from build123d import *

# Parameters (mm, degrees)
F0_W     = 120
F0_H     = 40
F1_DEPTH = 12.5
F3_DEPTH = 9.7
F4_W     = 110
F4_H     = 10.5
F5_DEPTH = 30
F6_W     = 110
F6_H     = 1.62
F7_DEPTH = 3.6
F8_R     = 0.5


with BuildPart() as f1:
    # F0 (on Front) → F1 (new body)
    with BuildSketch(Plane.XZ):
        Rectangle(F0_W, F0_H)
    extrude(amount=F1_DEPTH)

    # F2 (on face) → F3 (join)
    with BuildSketch(Plane(origin=(0, 0, 0), x_dir=(-1, 0, 0), z_dir=(0, 1, 0))):
        with BuildLine():
            Line((-25, -10), (25, -10))
            ThreePointArc((25, -10), (28.5355339059, -8.5355339059), (30, -5))
            Line((30, -5), (30, 5))
            ThreePointArc((30, 5), (28.5355339059, 8.5355339059), (25, 10))
            Line((25, 10), (-25, 10))
            ThreePointArc((-25, 10), (-28.5355339059, 8.5355339059), (-30, 5))
            Line((-30, 5), (-30, -5))
            ThreePointArc((-30, -5), (-28.5355339059, -8.5355339059), (-25, -10))
        make_face()
    extrude(amount=F3_DEPTH)

    # F4 (on face) → F5 (cut)
    with BuildSketch(Plane(origin=(0, 0, -20), x_dir=(1, 0, 0), z_dir=(0, 0, -1))):
        with Locations((0, 7.25)):
            Rectangle(F4_W, F4_H)
    extrude(amount=-F5_DEPTH, mode=Mode.SUBTRACT)

    # F6 (on face) → F7 (join)
    with BuildSketch(Plane(origin=(0, 0, 10), x_dir=(1, 0, 0), z_dir=(0, 0, -1))):
        with Locations((0, 9.67)):
            Rectangle(F6_W, F6_H)
    extrude(amount=F7_DEPTH)

    # F8
    f8_edges = [f1.edges().sort_by_distance(p)[0] for p in [
        (0, 9.7, -10),
        (0, -2, -20),
        (55, -7.25, -20),
        (55, -12.5, -5),
        (0, -12.5, 10),
        (-55, -12.5, -5),
        (-55, -7.25, -20),
        (57.5, -12.5, -20),
        (60, -12.5, 0),
        (0, -12.5, 20),
        (-60, -12.5, 0),
        (-57.5, -12.5, -20),
        (60, -6.25, -20),
        (60, -6.25, 20),
        (-60, -6.25, 20),
        (-60, -6.25, -20),
        (-60, 0, 0),
        (0, 0, 20),
        (0, 0, -20),
        (60, 0, 0),
    ]]
    fillet(f8_edges, radius=F8_R)


solid = f1.part
The listing builds one solid part. Answer for the finished solid, in the listing's coordinates (mm). A direction names the side the tool comes from. Round coordinates to 2 decimals unless told otherwise and drop trailing zeros. Write each loop counter-clockwise with the first axis right and the second up, starting at its lowest first coordinate (ties: lowest second). Pieces come first, ordered by that corner, then holes. Notation, with made-up numbers: (81.25, 67.25) - (118.25, 67.25) arc R14 ccw to (118.25, 71.25) - close; hole circle Ø5 at (-39.5, 56). An arc over 180 degrees is marked (long way). Use one line per item in the form item = value. Start each with the question number.
Item 1: A cutting plane is placed at D-D (y = 2.5). Write down the section's boundary in (x, z).
Item 2: Determine the mould class of faces 5 (the cylindrical face through (-28, 5, -9)), 6 (the flat face through (60, -6, 0)), 7 (the flat face through (-55, -7, -5)) for opening direction X: +X half, -X half, draft (parallel to the pull), parting line (faces both ways), or undercut.
Item 3: A tool of negligible diameter and unlimited length cuts with its end or side. For faces 1 (the flat face through (0, 5, -10)), 2 (the flat face through (-30, 5, 0)), 3 (the flat face through (-1, -10.48, 8)), 4 (the flat face through (-1, -5, 10)), from which of +Z, -Z, +X, -X, +Y, -Y can it reach the whole face along a straight path? Write none if from no direction.
Item 4: A cutting plane is placed at A-A (y = -7). Write down the section's boundary in (x, z).
Item 5: A cutting plane is placed at B-B (z = -1.5). Write down the section's boundary in (x, y), plus the area to 3 significant figures.
Item 6: A cutting plane is placed at C-C (x = 46). Write down the section's boundary in (y, z), plus the area to 3 significant figures.
Item 7: Flat-ended cylindrical pins translate along their axes: pin 1 Ø0.5 at (x, y) = (-23, -11.5) entering from -Z; pin 2 Ø4 at (x, y) = (-11, 7) entering from -Z; pin 3 Ø6 at (y, z) = (5.5, -14) entering from +X; pin 4 Ø5 at (x, z) = (42.5, -4) entering from -Y. Find the tip coordinate at first contact, or state that the pin passes through.
Item 8: Find the intervals of material crossed by line 1 (X direction, y = -10, z = 6); line 2 (X direction, y = 1.5, z = 5); line 3 (Z direction, x = -24, y = 2), in increasing order. Write a range as [from, to].
The answers:
q1.outline = (-30, -5) arc R5 ccw to (-25, -10) - (25, -10) arc R5 ccw to (30, -5) - (30, 5) arc R5 ccw to (25, 10) - (-25, 10) arc R5 ccw to (-30, 5) - close
q2.face_5 = -X half
q2.face_6 = +X half
q2.face_7 = undercut
q3.face_1 = -Z, +X, -X, +Y
q3.face_2 = +Z, -Z, -X, +Y
q3.face_3 = -Z, -Y
q3.face_4 = -Z
q4.outline = (-60, -19.5) arc R0.5 ccw to (-59.5, -20) - (-55.5, -20) arc R0.5 ccw to (-55, -19.5) - (-55, 10) - (55, 10) - (55, -19.5) arc R0.5 ccw to (55.5, -20) - (59.5, -20) arc R0.5 ccw to (60, -19.5) - (60, 19.5) arc R0.5 ccw to (59.5, 20) - (-59.5, 20) arc R0.5 ccw to (-60, 19.5) - close
q5.outline = (-60, -12) arc R0.5 ccw to (-59.5, -12.5) - (-55.5, -12.5) arc R0.5 ccw to (-55, -12) - (-55, -2) - (55, -2) - (55, -12) arc R0.5 ccw to (55.5, -12.5) - (59.5, -12.5) arc R0.5 ccw to (60, -12) - (60, -0.5) arc R0.5 ccw to (59.5, 0) - (30, 0) - (30, 9.2) arc R0.5 ccw to (29.5, 9.7) - (-29.5, 9.7) arc R0.5 ccw to (-30, 9.2) - (-30, 0) - (-59.5, 0) arc R0.5 ccw to (-60, -0.5) - close
q5.area = 927 mm^2
q6.outline = (-12.5, 10.5) arc R0.5 ccw to (-12, 10) - (-10.48, 10) - (-10.48, 6.4) - (-8.86, 6.4) - (-8.86, 10) - (-2, 10) - (-2, -19.5) arc R0.5 ccw to (-1.5, -20) - (-0.5, -20) arc R0.5 ccw to (0, -19.5) - (0, 19.5) arc R0.5 ccw to (-0.5, 20) - (-12, 20) arc R0.5 ccw to (-12.5, 19.5) - close
q6.area = 191 mm^2
q7.pin_1 = 10
q7.pin_2 = -10
q7.pin_3 = through
q7.pin_4 = -2
q8.line_1 = [-60, -55], [55, 60]
q8.line_2 = [-30, 30]
q8.line_3 = [-10, 10]
